Geometry: see drawing. Coordinates: mm, zero at the bounding-box minimum. Coordinates: 2 decimals unless noted, no trailing zeros. Write each loop counter-clockwise with the first axis right and the second up, starting at its lowest first coordinate (ties: lowest second). Pieces come first, ordered by that corner, then holes. Notation, with made-up numbers: M 69.25,-11 L 101.25,-11 A6 cw 101.25,-5 Z; hole C -13.5,87.5 d8. An arc over 180 degrees is marked long. One line per item, written item: value. Start each with the question number.
Item 1: Pin query (flat end, axial travel): P1, Ø0.9, axis at x = 3, y = 1.5, coming from the -Z side; P2, Ø1.5, axis at x = 19.5, y = 1, coming from the +Z side; P3, Ø0.9, axis at y = 2, z = 156.5, coming from the +X side; P4, Ø3, axis at x = 115, z = 34, coming from the -Y side. Return the tip coordinate at first contact, or that it passes through.
Item 2: Cut plane C-C, the plane x = 28. Output: boundary loops of the cut face in (y, z), then the cut area to 3 significant figures.
Item 3: Cut plane A-A, the plane z = 143.5. Output: boundary loops of the cut face in (x, y).
Item 4: Cut plane B-B, the plane y = 2.5. State how many separate pieces and enclosed holes the cut face has, then the cut area to 3 significant figures.
Item 5: Ray query, L1, parallel to X at y = 1.9, z = 149.5; L2, parallel to Z at x = 170.5, y = 0.5; L3, parallel to Z at x = 36.5, y = 0.35. Return the intervals inside material, ascending. Write a range as from..to.
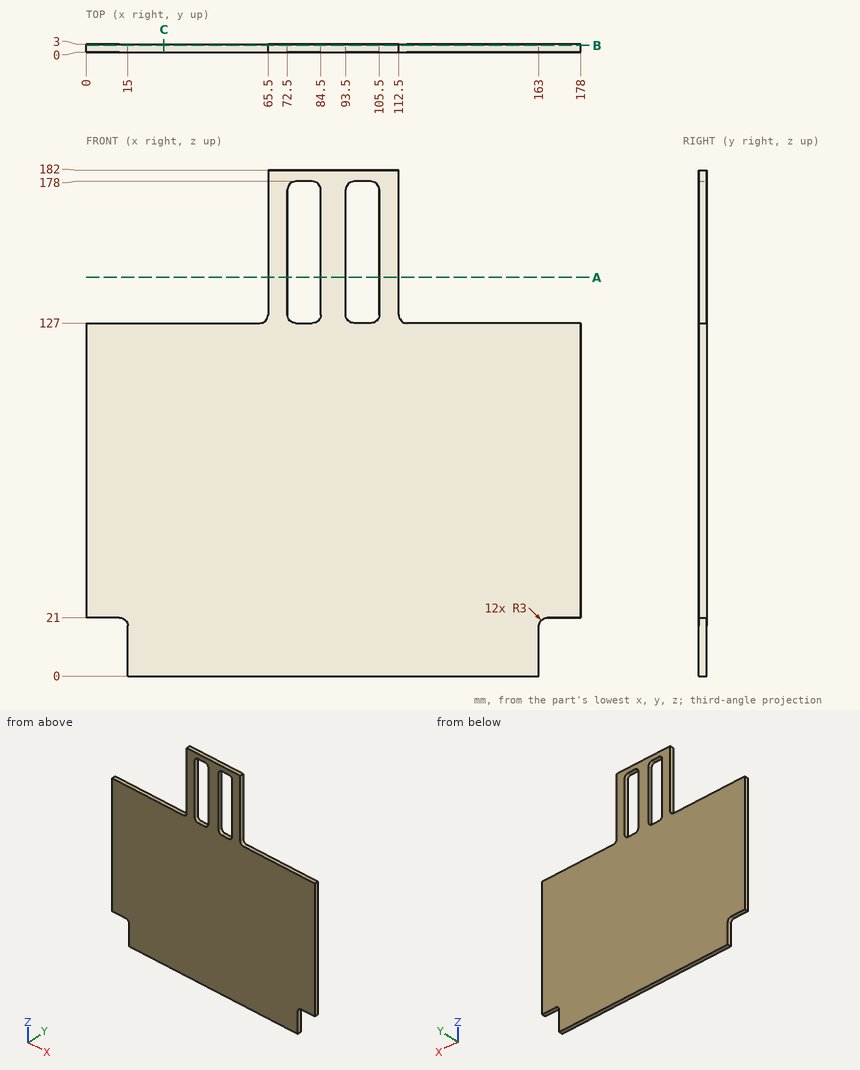
From the geometry:
1. P1: stops at z = 21
1. P2: stops at z = 127
1. P3: stops at x = 112.5
1. P4: stops at y = 0
2. outline: M 0,0 L 3,0 L 3,127 L 0,127 Z
2. area: 381 mm²
3. outline: M 65.5,0 L 72.5,0 L 72.5,3 L 65.5,3 Z; M 84.5,0 L 93.5,0 L 93.5,3 L 84.5,3 Z; M 105.5,0 L 112.5,0 L 112.5,3 L 105.5,3 Z
4. separate pieces: 1
4. enclosed holes: 2
4. area: 23,400 mm²
5. L1: x = 65.5..72.5, 84.5..93.5, 105.5..112.5
5. L2: z = 21..127
5. L3: z = 0..127
